CAD build for the part. Positions are in the model's coordinates, mm. Round coordinates to 2 decimals unless told otherwise and drop trailing zeros. Loops run counter-clockwise (first coordinate to the right, second up) from the corner with the lowest first, then second, coordinate; pieces in that order, holes last. Notation, with made-up numbers: M 10.25,71 L 27.25,71 A12 ccw 27.25,90 Z; hole C 58,5 d11. An arc over 180 degrees is marked long. Use one line per item in the form item = value.
from build123d import *

# Parameters (mm, degrees)
BOSS_EXTRUDE1_DEPTH = 3
SKETCH2_R           = 2.5
CUT_EXTRUDE1_DEPTH  = 3


with BuildPart() as part:
    # Sketch1 → Boss-Extrude1 (new body)
    with BuildSketch(Plane.XY):
        Polygon((0, 60), (20, 60), (60, 20), (60, 0), (0, 0), align=None)
    extrude(amount=-BOSS_EXTRUDE1_DEPTH)

    # Sketch2 → Cut-Extrude1 (cut)
    with BuildSketch(Plane.XY):
        with Locations((10, 10)):
            Circle(SKETCH2_R)
        with Locations((30, 10)):
            Circle(SKETCH2_R)
        with Locations((50, 10)):
            Circle(SKETCH2_R)
        with Locations((10, 30)):
            Circle(SKETCH2_R)
        with Locations((10, 50)):
            Circle(SKETCH2_R)
    extrude(amount=-CUT_EXTRUDE1_DEPTH, mode=Mode.SUBTRACT)


solid = part.part
1. Probe line 1 along Y through (x, z) = (10, -2.1); line 2 along Y through (x, z) = (12, -2.8); line 3 along Y through (x, z) = (50, -1.6). List the from-to ranges inside material, lowest first. Write a range as from..to.
Completed:
line_1 = 0..7.5, 12.5..27.5, 32.5..47.5, 52.5..60
line_2 = 0..8.5, 11.5..28.5, 31.5..48.5, 51.5..60
line_3 = 0..7.5, 12.5..30
2. Cut at A-A on x = 50. Write the cut outline in (y, z).
Completed:
outline = M 0,-3 L 7.5,-3 L 7.5,0 L 0,0 Z; M 12.5,-3 L 30,-3 L 30,0 L 12.5,0 Z
3. Pull direction Y, two halves, no side cores. Call faces 1 (the face through (10, 60, -1)), 2 (the face through (60, 10, -1)), 3 (the face through (29.46, 7.56, -1.48)): +Y half, -Y half, draft (parallel to the pull), parting line (faces both ways), or undercut.
Completed:
face_1 = +Y half
face_2 = draft
face_3 = undercut
4. Cut at D-D on y = 10. Write the cut outline in (x, z), and give its area (3 significant figures).
Completed:
outline = M 0,-3 L 7.5,-3 L 7.5,0 L 0,0 Z; M 12.5,-3 L 27.5,-3 L 27.5,0 L 12.5,0 Z; M 32.5,-3 L 47.5,-3 L 47.5,0 L 32.5,0 Z; M 52.5,-3 L 60,-3 L 60,0 L 52.5,0 Z
area = 135 mm2
5. Cut at C-C on z = -1.7. Write the cut outline in (x, y).
Completed:
outline = M 0,0 L 60,0 L 60,20 L 20,60 L 0,60 Z; hole C 10,10 d5; hole C 10,30 d5; hole C 10,50 d5; hole C 30,10 d5; hole C 50,10 d5
6. Drop a flat-ended pin along its axis: P1, Ø4, axis at x = 30, y = 10, coming from the +Z side. Give the stop position or say it passes through.
Completed:
P1 = through
